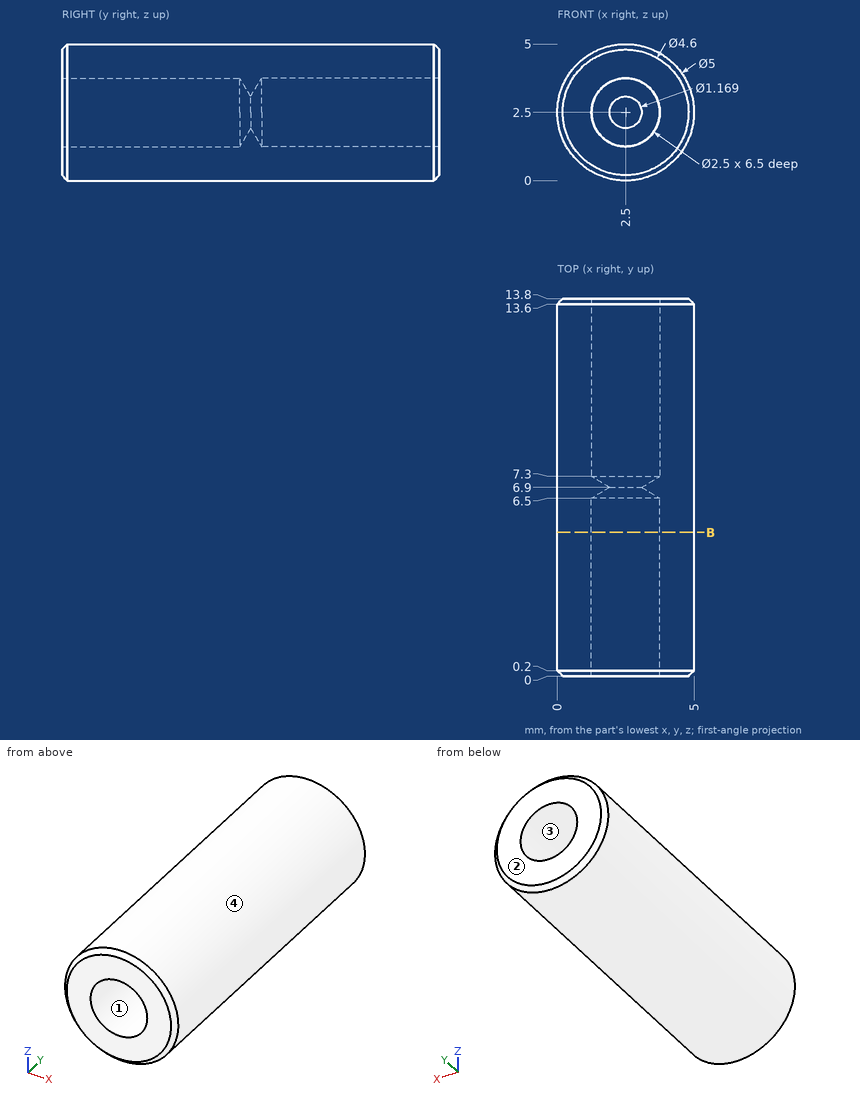
Geometry: see drawing. Coordinates: mm, zero at the bounding-box minimum. Give positions to 0.01 mm unless a question says otherwise; leave off trailing zeros. Write each loop counter-clockwise with the first axis right and the second up, starting at its lowest first coordinate (ties: lowest second). Pieces come first, ordered by that corner, then holes. Notation, with made-up numbers: M 72,-15.75 L 96,-15.75 A30 cw 96,19.25 Z; hole C -9,2.25 d3. An arc over 180 degrees is marked long. Answer as a JSON object with one key per item and string values.
Q1. Contact query for flat-ended pins moving along their axis: P1, Ø2, axis at x = 2.5, z = 3.5, coming from the +Y side; P2, Ø2, axis at x = 2.5, z = 2.5, coming from the +Y side; P3, Ø1.5, axis at x = 2.5, z = 2.5, coming from the +Y side. Output: stop coordinate, or through.
Geometry check:
{"P1": "stops at y = 13.8", "P2": "stops at y = 7.15", "P3": "stops at y = 7"}
Q2. Mould query, pull axis X, two halves, no side actions, for the marked faces 1, 2, 3 and 4. Classes: +X half, -X half, draft (parallel to the pull), parting line (faces both ways), or undercut.
Geometry check:
{"face 1": "undercut", "face 2": "draft", "face 3": "undercut", "face 4": "parting line"}
Q3. Ray query, line 1 along X through (y, z) = (0.75, 1.95); line 2 along X through (y, z) = (3.25, 2.95) (1 decimal). Return the intervals inside material, ascending.
Geometry check:
{"line 1": "x = 0.06 to 1.38, 3.62 to 4.94", "line 2": "x = 0 to 1.3, 3.7 to 5"}
Q4. Cut plane B-B, the plane y = 5.25. Return the cut outline in (x, z), then the cut area to 3 significant figures.
Geometry check:
{"outline": "C 2.5,2.5 d5; hole C 2.5,2.5 d2.5", "area": "14.7 mm^2"}
